Check sheet for the drawn part. Datum: minimum x, y, z corner. Units: mm. A direction names the side the tool comes from. Round coordinates to 2 decimals unless told otherwise and drop trailing zeros. Write each loop counter-clockwise with the first axis right and the second up, starting at its lowest first coordinate (ties: lowest second). Pieces come first, ordered by that corner, then holes. Notation, with made-up numbers: M 23,83.25 L 59,83.25 A19 cw 59,97.25 Z; hole C 29.5,-23.75 d5. An arc over 180 degrees is marked long. Answer in a Markdown table with one row per item. Add a question column.
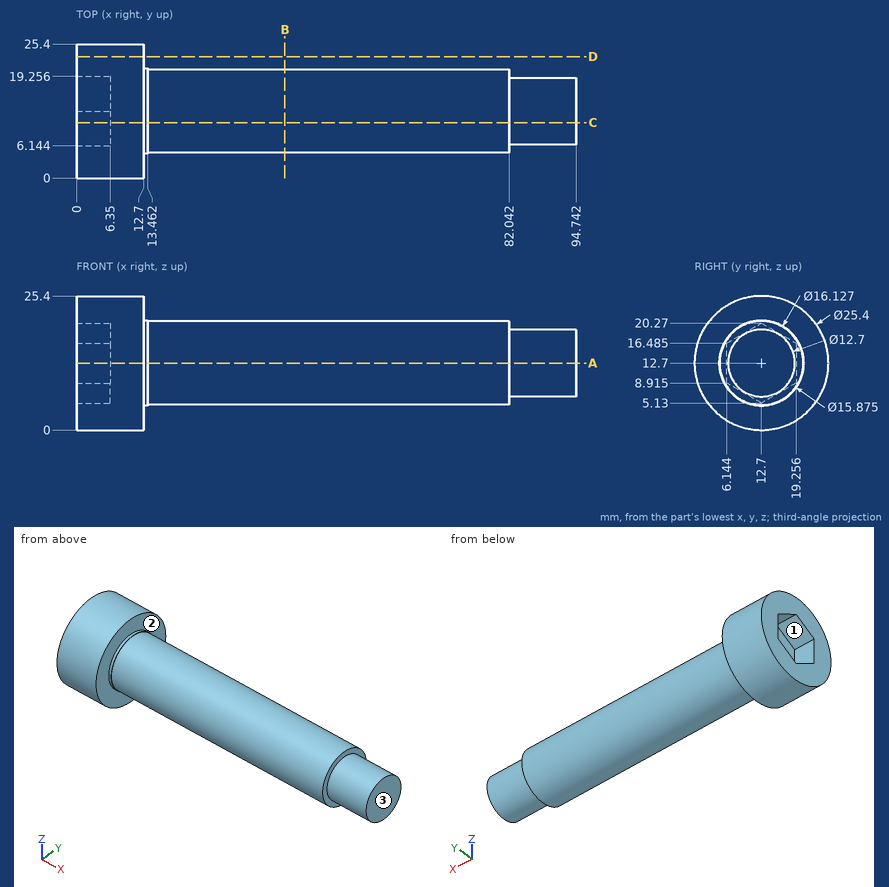
Item 1: Section check D-D, the plane y = 23. Record the boundary of the cut face in (x, z), and give its area (3 significant figures).
Item 2: Section check C-C, the plane y = 10.5. Record the boundary of the cut face in (x, z), and give its area (3 significant figures).
Item 3: Section check B-B, the plane x = 39.5. Record the boundary of the cut face in (y, z) (1 decimal), and give its area (3 significant figures).
Item 4: Scan lines: probe 1 along X at (y, z) = (20, 16); probe 2 along X at (y, z) = (12.25, 2.5); probe 3 along Z at (x, y) = (51, 13.25). Record each from-to range of solid material in increasing order. Write a range as from..to.
Item 5: Section check A-A, the plane z = 12.7. Record the boundary of the cut face in (x, y).
Item 6: Gauge pin test, flat ends, axial feed: pin 1 Ø1.5 at (y, z) = (22, 10.5) entering from +X; pin 2 Ø2 at (x, z) = (73.5, 20) entering from +Y; pin 3 Ø4 at (x, z) = (57, 6.5) entering from +Y (1 decimal). Record the tip position at first contact, or that the pin passes through.
Item 7: Access from +Z, -Z, +X, -X, +Y, -Y to the whole of each face (thin tool, end or side, straight path). Record for the marked faces 1, 2 and 3.
Result sheet:
| question | item | result |
|---|---|---|
| 1 | outline | M 0,5.27 L 12.7,5.27 L 12.7,20.13 L 0,20.13 Z |
| 1 | area | 189 mm^2 |
| 2 | outline | M 0,0.19 L 12.7,0.19 L 12.7,4.94 L 13.46,4.94 L 13.46,5.07 L 82.04,5.07 L 82.04,6.74 L 94.74,6.74 L 94.74,18.66 L 82.04,18.66 L 82.04,20.33 L 13.46,20.33 L 13.46,20.46 L 12.7,20.46 L 12.7,25.21 L 0,25.21 L 0,19 L 6.35,19 L 6.35,6.4 L 0,6.4 Z |
| 2 | area | 1,450 mm^2 |
| 3 | outline | C 12.7,12.7 d15.9 |
| 3 | area | 198 mm^2 |
| 4 | probe 1 | x = 0..13.46 |
| 4 | probe 2 | x = 0..12.7 |
| 4 | probe 3 | z = 4.78..20.62 |
| 5 | outline | M 0,0 L 12.7,0 L 12.7,4.64 L 13.46,4.64 L 13.46,4.76 L 82.04,4.76 L 82.04,6.35 L 94.74,6.35 L 94.74,19.05 L 82.04,19.05 L 82.04,20.64 L 13.46,20.64 L 13.46,20.76 L 12.7,20.76 L 12.7,25.4 L 0,25.4 L 0,19.26 L 6.35,19.26 L 6.35,6.14 L 0,6.14 Z |
| 6 | pin 1 | stops at x = 12.7 |
| 6 | pin 2 | stops at y = 17.53 |
| 6 | pin 3 | stops at y = 19.4 |
| 7 | face 1 | -X |
| 7 | face 2 | +X |
| 7 | face 3 | +Z, -Z, +X, +Y, -Y |
